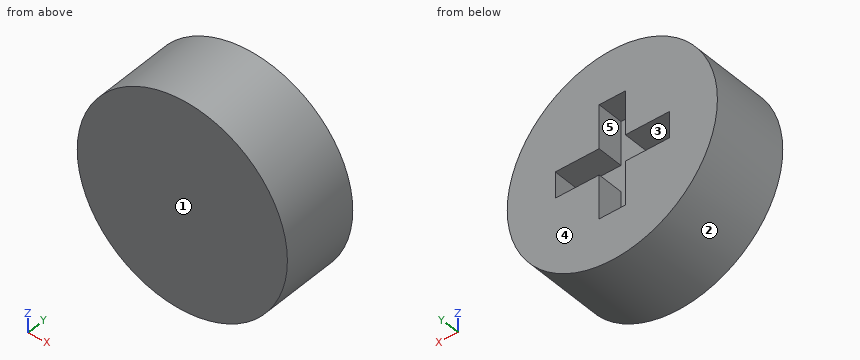
from build123d import *

# Parameters (mm, degrees)
F0_R     = 5.08
F1_DEPTH = 3.81
F2_W     = 2.1238556986
F2_H     = 1.27
F2_W_2   = 1.27
F2_H_2   = 2.1238556986
F3_DEPTH = 1.27


with BuildPart() as f1:
    # F0 (on Front) → F1 (new body)
    with BuildSketch(Plane.XZ):
        Circle(F0_R)
    extrude(amount=F1_DEPTH)

    # F2 (on Front) → F3 (cut)
    with BuildSketch(Plane.XZ):
        with Locations((-1.6969278493, 0)):
            Rectangle(F2_W, F2_H)
        Rectangle(F2_W_2, F2_H)
        with Locations((0, 1.6969278493)):
            Rectangle(F2_W_2, F2_H_2)
        with Locations((1.6969278493, 0)):
            Rectangle(F2_W, F2_H)
        with Locations((0, -1.6969278493)):
            Rectangle(F2_W_2, F2_H_2)
    extrude(amount=F3_DEPTH, mode=Mode.SUBTRACT)


solid = f1.part
CAD build for the part. Positions are in the model's coordinates, mm. Face numbers are marked on the shaded views. A direction names the side the tool comes from. Round coordinates to 2 decimals unless told otherwise and drop trailing zeros. Write each loop counter-clockwise with the first axis right and the second up, starting at its lowest first coordinate (ties: lowest second). Pieces come first, ordered by that corner, then holes.
(1) Slice it at B-B, the plane x = 0. Write the cut outline in (y, z).
(2) Probe line 1 along Z through (x, y) = (0, -1.1); line 2 along Z through (x, y) = (-1, -0.45) (3 decimals); line 3 along X through (y, z) = (-1, 0.5). List the from-to ranges inside material, lowest first.
(3) Drop flat-ended pins along their axis: P1, Ø1.4, axis at y = -0.5, z = 1, coming from the -X side; P2, Ø0.6, axis at y = -0.5, z = 1.5, coming from the +X side; P3, Ø1.5, axis at x = 2, y = -1, coming from the +Z side. Give the stop position or say it passes through.
(4) Mould opens along X. For the marked faces 1, 2 and 3 say: pulls with the +X half, pulls with the -X half, needs draft (parallel to the pull), parting line crosses it, or undercut.
(5) Slice it at C-C, the plane z = 0. Write the cut outline in (x, y), and give its area (3 significant figures).
(6) Slice it at A-A, the plane y = -0.45. Write the cut outline in (x, z) (3 decimals), and give its area (3 significant figures).
(7) Slice it at D-D, the plane y = -1.65. Write the cut outline in (x, z), and give its area (3 significant figures).
(8) 3-axis set-ups, long thin cutter, end or side, ignore diameter. For the marked faces 4 and 5: which of +Z, -Z, +X, -X, +Y, -Y reach the whole face in a straight line?
From the geometry:
1. outline: (-3.81, -5.08) - (0, -5.08) - (0, -2.76) - (-1.27, -2.76) - (-1.27, 2.76) - (0, 2.76) - (0, 5.08) - (-3.81, 5.08) - close
2. line 1: z = -5.08 to -2.76, 2.76 to 5.08
2. line 2: z = -4.981 to -0.635, 0.635 to 4.981
2. line 3: x = -5.06 to -2.76, 2.76 to 5.06
3. P1: stops at x = -5.07
3. P2: stops at x = 4.94
3. P3: stops at z = 4.92
4. face 1: needs draft
4. face 2: parting line crosses it
4. face 3: undercut
5. outline: (-5.08, -3.81) - (5.08, -3.81) - (5.08, 0) - (2.76, 0) - (2.76, -1.27) - (-2.76, -1.27) - (-2.76, 0) - (-5.08, 0) - close
5. area: 31.7 mm2
6. outline: circle Ø10.16 at (0, 0); hole (-2.759, -0.635) - (-0.635, -0.635) - (-0.635, -2.759) - (0.635, -2.759) - (0.635, -0.635) - (2.759, -0.635) - (2.759, 0.635) - (0.635, 0.635) - (0.635, 2.759) - (-0.635, 2.759) - (-0.635, 0.635) - (-2.759, 0.635) - close
6. area: 68.7 mm2
7. outline: circle Ø10.16 at (0, 0)
7. area: 81.1 mm2
8. face 4: +Z, -Z, +X, -X, +Y
8. face 5: +Y
